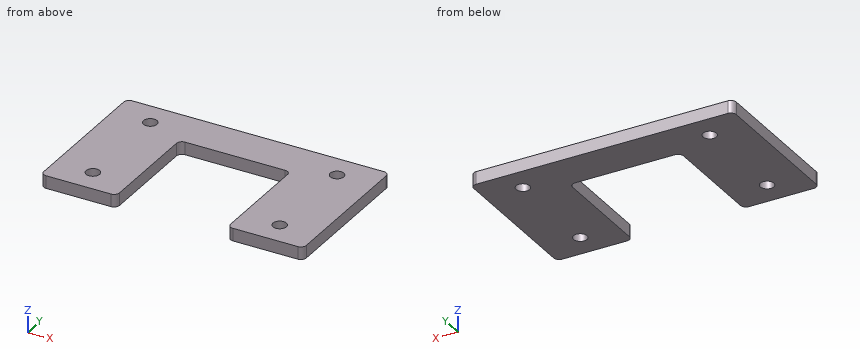
```python
from build123d import *

# Parameters (mm, degrees)
SKETCH1_R           = 2.693094888
BOSS_EXTRUDE1_DEPTH = 5


with BuildPart() as part:
    # Sketch1 → Boss-Extrude1 (new body)
    with BuildSketch(Plane.XY):
        with BuildLine():
            Line((326.218649089, 421.822340311), (351.909697268, 421.822340311))
            ThreePointArc((351.909697268, 421.822340311), (353.433141794, 422.453371695), (354.064173178, 423.976816221))
            Line((354.064173178, 423.976816221), (354.064173178, 463.6678644))
            ThreePointArc((354.064173178, 463.6678644), (354.695204563, 465.191308926), (356.218649089, 465.822340311))
            Line((356.218649089, 465.822340311), (395.909699459, 465.822340311))
            ThreePointArc((395.909699459, 465.822340311), (397.433143985, 465.191308926), (398.064175369, 463.6678644))
            Line((398.064175369, 463.6678644), (398.064175369, 423.976816221))
            ThreePointArc((398.064175369, 423.976816221), (398.695206753, 422.453371695), (400.218651279, 421.822340311))
            Line((400.218651279, 421.822340311), (425.909697268, 421.822340311))
            ThreePointArc((425.909697268, 421.822340311), (427.433141794, 422.453371695), (428.064173178, 423.976816221))
            Line((428.064173178, 423.976816221), (428.064173178, 479.6678644))
            ThreePointArc((428.064173178, 479.6678644), (427.433141794, 481.191308926), (425.909697268, 481.822340311))
            Line((425.909697268, 481.822340311), (326.218649089, 481.822340311))
            ThreePointArc((326.218649089, 481.822340311), (324.695204563, 481.191308926), (324.064173178, 479.6678644))
            Line((324.064173178, 479.6678644), (324.064173178, 423.976816221))
            ThreePointArc((324.064173178, 423.976816221), (324.695204563, 422.453371695), (326.218649089, 421.822340311))
        make_face()
        with Locations((339.064173178, 471.822340311)):
            Circle(SKETCH1_R, mode=Mode.SUBTRACT)
        with Locations((339.064173178, 431.822340311)):
            Circle(SKETCH1_R, mode=Mode.SUBTRACT)
        with Locations((413.064174274, 431.822340311)):
            Circle(SKETCH1_R, mode=Mode.SUBTRACT)
        with Locations((413.064174274, 471.822340311)):
            Circle(SKETCH1_R, mode=Mode.SUBTRACT)
    extrude(amount=-BOSS_EXTRUDE1_DEPTH)


solid = part.part
```
Can you work these out from the model? Positions are in its coordinate system, mm. Give positions to 0.01 mm unless a question says otherwise; leave off trailing zeros. Order: outer loops, then holes, each group sorted by start corner. A loop starts at its lowest first (then second) coordinate and runs counter-clockwise, first axis right, second up. Notation, with made-up numbers: (86.5, 14.5) - (103.5, 14.5) arc R14 ccw to (103.5, 36.5) - close; hole circle Ø11 at (26.5, -18). An arc over 180 degrees is marked (long way). Use a Markdown table: item, result. Add a question column.
Q1. Please list where these lines run through material, in increasing order: line 1 along X through (y, z) = (469.5, -3.6); line 2 along X through (y, z) = (437, -3.5); line 3 along Y through (x, z) = (338, -2.1).
Q2. If we section it at C-C on y = 473.5: Write out the boundary of the cut face in (x, z), plus the area to 3 significant figures.
Q3. If we section it at A-A on y = 447: Write out the boundary of the cut face in (x, z), plus the area to 3 significant figures.
Q4. I'm going to push a flat-ended pin straight in: pin 1 (1.5 mm diameter, centred on x = 385, z = -2, fed in from -Y). Where does the tip first touch, or does it pass through?
Q5. If we section it at B-B on z = -3.45: Write out the boundary of the cut face in (x, y).
Answers follow:
| question | item | result |
|---|---|---|
| 1 | line 1 | x = 324.06 to 337.7, 340.43 to 411.7, 414.43 to 428.06 |
| 1 | line 2 | x = 324.06 to 354.06, 398.06 to 428.06 |
| 1 | line 3 | y = 421.82 to 429.35, 434.3 to 469.35, 474.3 to 481.82 |
| 2 | outline | (324.06, -5) - (336.96, -5) - (336.96, 0) - (324.06, 0) - close; (341.17, -5) - (410.96, -5) - (410.96, 0) - (341.17, 0) - close; (415.17, -5) - (428.06, -5) - (428.06, 0) - (415.17, 0) - close |
| 2 | area | 478 mm^2 |
| 3 | outline | (324.06, -5) - (354.06, -5) - (354.06, 0) - (324.06, 0) - close; (398.06, -5) - (428.06, -5) - (428.06, 0) - (398.06, 0) - close |
| 3 | area | 300 mm^2 |
| 4 | pin 1 | stops at y = 465.82 |
| 5 | outline | (324.06, 423.98) arc R2.15 ccw to (326.22, 421.82) - (351.91, 421.82) arc R2.15 ccw to (354.06, 423.98) - (354.06, 463.67) arc R2.15 cw to (356.22, 465.82) - (395.91, 465.82) arc R2.15 cw to (398.06, 463.67) - (398.06, 423.98) arc R2.15 ccw to (400.22, 421.82) - (425.91, 421.82) arc R2.15 ccw to (428.06, 423.98) - (428.06, 479.67) arc R2.15 ccw to (425.91, 481.82) - (326.22, 481.82) arc R2.15 ccw to (324.06, 479.67) - close; hole circle Ø5.39 at (339.06, 431.82); hole circle Ø5.39 at (339.06, 471.82); hole circle Ø5.39 at (413.06, 431.82); hole circle Ø5.39 at (413.06, 471.82) |
